```python
from build123d import *

# Parameters (mm, degrees)
SKETCH1_W                = 13
SKETCH1_H                = 8.15
BOSS_EXTRUDE1_DEPTH      = 9.5
SKETCH2_R                = 2.9
BOSS_EXTRUDE2_DEPTH      = 8.5
BOSS_EXTRUDE3_DEPTH      = 1.5
BOSS_EXTRUDE3_DEPTH_BACK = 1.5
SKETCH4_W                = 10
SKETCH4_H                = 2
BOSS_EXTRUDE4_DEPTH      = 3.85
CUT_EXTRUDE1_DEPTH       = 21.027621551
CUT_EXTRUDE1_DEPTH_BACK  = 21.027621551
SKETCH5_W                = 1.66278511
SKETCH5_H                = 3.85


with BuildPart() as part:
    # Sketch1 → Boss-Extrude1 (new body)
    with BuildSketch(Plane(origin=(0, 0, 0), x_dir=(1, 0, 0), z_dir=(0, 1, 0))):
        Rectangle(SKETCH1_W, SKETCH1_H)
    extrude(amount=-BOSS_EXTRUDE1_DEPTH)

    # Sketch2 → Boss-Extrude2 (add)
    with BuildSketch(Plane(origin=(0, 0, 0), x_dir=(1, 0, 0), z_dir=(0, 1, 0))):
        with Locations(Location((0, 0, 0), (0, 0, 270))):
            Circle(SKETCH2_R)
    extrude(amount=BOSS_EXTRUDE2_DEPTH)

    # Sketch3 → Boss-Extrude3 (add, two sides: drawn at the far end of the back side and taken through both)
    with BuildSketch(Plane.XY.offset(-BOSS_EXTRUDE3_DEPTH_BACK)):
        Polygon((3.25, 18.5), (-3.25, 18.5), (-1.5, 8.5), (1.5, 8.5), align=None)
    extrude(amount=BOSS_EXTRUDE3_DEPTH + BOSS_EXTRUDE3_DEPTH_BACK)

    # Sketch4 → Boss-Extrude4 (add)
    with BuildSketch(Plane.XZ.offset(9.5)):
        Rectangle(SKETCH4_W, SKETCH4_H)
    extrude(amount=BOSS_EXTRUDE4_DEPTH)

    # Sketch5 → Cut-Extrude1 (cut, two sides: drawn at the far end of the back side and taken through both)
    with BuildSketch(Plane.XY.offset(-CUT_EXTRUDE1_DEPTH_BACK)):
        with Locations((-2.017335511, -11.425)):
            Rectangle(SKETCH5_W, SKETCH5_H)
        with Locations((2.017335511, -11.425)):
            Rectangle(SKETCH5_W, SKETCH5_H)
    extrude(amount=CUT_EXTRUDE1_DEPTH + CUT_EXTRUDE1_DEPTH_BACK, mode=Mode.SUBTRACT)


solid = part.part
```
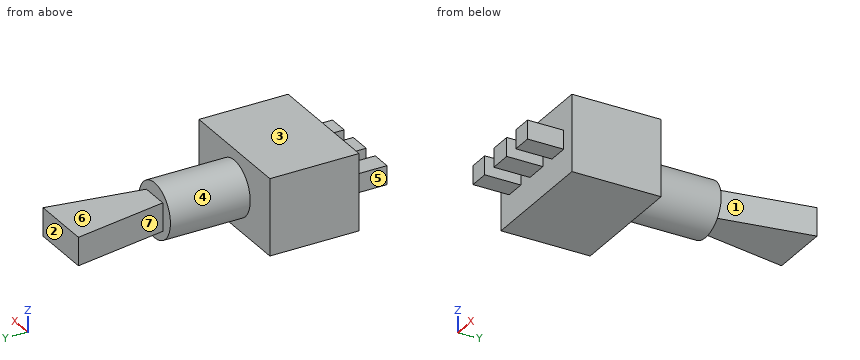
Verification items for the finished model (mm, model axes). Face numbers are marked on the shaded views. A direction names the side the tool comes from. Coordinates: 2 decimals unless noted, no trailing zeros. Loops run counter-clockwise (first coordinate to the right, second up) from the corner with the lowest first, then second, coordinate; pieces in that order, holes last. Notation, with made-up numbers: (64.25, 6.5) - (70.25, 6.5) arc R27 ccw to (70.25, 37.5) - close; hole circle Ø7 at (36, 55). An arc over 180 degrees is marked (long way). Answer as a JSON object with one key per item and string values.
(1) Cross-section at D-D, the plane y = 16. Record the boundary of the cut face in (x, z).
Response:
{"outline": "(-2.81, -1.5) - (2.81, -1.5) - (2.81, 1.5) - (-2.81, 1.5) - close"}
(2) Access from +Z, -Z, +X, -X, +Y, -Y to the whole of each face (thin tool, end or side, straight path). Record for the marked faces 4, 5, 6 and 7.
Response:
{"face 4": "none", "face 5": "+Z, -Z, -X, -Y", "face 6": "+Z, +X, -X, +Y", "face 7": "+Z, -Z, -X"}
(3) Scan lines: line 1 along Y through (x, z) = (0.5, 2.5); line 2 along Z through (x, y) = (2.25, 14); line 3 along Y through (x, z) = (5, 1). Record each from-to range of solid material in increasing order.
Response:
{"line 1": "y = -9.5 to 8.5", "line 2": "z = -1.5 to 1.5", "line 3": "y = -9.5 to 0"}
(4) Cross-section at C-C, the plane x = -2.5. Record the boundary of the cut face in (y, z) (3 decimals).
Response:
{"outline": "(-9.5, -4.075) - (0, -4.075) - (0, -1.47) - (8.5, -1.47) - (8.5, 1.47) - (0, 1.47) - (0, 4.075) - (-9.5, 4.075) - close; (14.214, -1.5) - (18.5, -1.5) - (18.5, 1.5) - (14.214, 1.5) - close"}
(5) Cross-section at B-B, the plane x = -4. Record the boundary of the cut face in (y, z) (3 decimals), then the cut area to 3 significant figures.
Response:
{"outline": "(-13.35, -1) - (-9.5, -1) - (-9.5, -4.075) - (0, -4.075) - (0, 4.075) - (-9.5, 4.075) - (-9.5, 1) - (-13.35, 1) - close", "area": "85.1 mm²"}
(6) Go/stop test with flat-tipped pins: pin 1 Ø1.5 at (x, z) = (5, 1.5) entering from +Y; pin 2 Ø2 at (x, y) = (-3.5, 5.5) entering from -Z; pin 3 Ø1.6 at (y, z) = (-12, 0) entering from +X. Record where each tip stops, or that it passes through.
Response:
{"pin 1": "stops at y = 0", "pin 2": "stops at z = -1.47", "pin 3": "stops at x = 5"}
(7) Mould release check, pull along Y, two halves, no side actions. Record for the marked faces 1, 2 and 3: pulls with the +Y half, pulls with the -Y half, needs draft (parallel to the pull), parting line crosses it, or undercut.
Response:
{"face 1": "undercut", "face 2": "pulls with the +Y half", "face 3": "needs draft"}
(8) Cross-section at A-A, the plane z = 0. Record the boundary of the cut face in (x, y).
Response:
{"outline": "(-6.5, -9.5) - (-5, -9.5) - (-5, -13.35) - (-2.85, -13.35) - (-2.85, -9.5) - (-1.19, -9.5) - (-1.19, -13.35) - (1.19, -13.35) - (1.19, -9.5) - (2.85, -9.5) - (2.85, -13.35) - (5, -13.35) - (5, -9.5) - (6.5, -9.5) - (6.5, 0) - (2.9, 0) - (2.9, 8.5) - (1.5, 8.5) - (3.25, 18.5) - (-3.25, 18.5) - (-1.5, 8.5) - (-2.9, 8.5) - (-2.9, 0) - (-6.5, 0) - close"}
